from build123d import *

# Parameters (mm, degrees)
F0_W     = 404
F0_H     = 145
F2_DEPTH = 3
F3_D     = 3.3
F3_DEPTH = 8.6
F3_TIP   = 0.9914200214
F1_R     = 1.5
F1_R_2   = 15
F1_R_3   = 1.75
F1_R_4   = 2.5
F1_W     = 55
F1_H     = 15
F4_DEPTH = 25


with BuildPart() as f2:
    # F0 (on Top) → F2 (new body)
    with BuildSketch(Plane.XY):
        with Locations((-14.1859020234, -7.6260944492)):
            Rectangle(F0_W, F0_H)
    extrude(amount=-F2_DEPTH)

    # F3
    with Locations(Plane.XY):
        with Locations((118.573140085, 24.8739055508), (158.573140085, 24.8739055508), (93.573140085, 24.8739055508), (53.573140085, 24.8739055508), (53.573140085, -40.1260944492), (93.573140085, -40.1260944492), (118.573140085, -40.1260944492), (158.573140085, -40.1260944492), (28.573140085, -40.1260944492), (-11.426859915, -40.1260944492), (-11.426859915, 24.8739055508), (28.573140085, 24.8739055508), (-35.926859915, 24.8739055508), (-80.926859915, 24.8739055508), (-80.926859915, -40.1260944492), (-35.926859915, -40.1260944492)):
            Hole(F3_D / 2, depth=F3_DEPTH)
            with Locations((0, 0, -(F3_DEPTH + F3_TIP / 2))):  # 118° drill point
                Cone(0, F3_D / 2, F3_TIP, mode=Mode.SUBTRACT)

    # F1 (on Top) → F4 (cut)
    with BuildSketch(Plane.XY):
        with BuildLine():
            Line((126.323140085, 12.4739055508), (150.823140085, 12.4739055508))
            ThreePointArc((150.823140085, 12.4739055508), (153.6515672098, 13.645478426), (154.823140085, 16.4739055508))
            Line((154.823140085, 16.4739055508), (154.823140085, 33.2739055508))
            ThreePointArc((154.823140085, 33.2739055508), (153.6515672098, 36.1023326755), (150.823140085, 37.2739055508))
            Line((150.823140085, 37.2739055508), (126.323140085, 37.2739055508))
            ThreePointArc((126.323140085, 37.2739055508), (123.4947129603, 36.1023326755), (122.323140085, 33.2739055508))
            Line((122.323140085, 33.2739055508), (122.323140085, 16.4739055508))
            ThreePointArc((122.323140085, 16.4739055508), (123.4947129603, 13.645478426), (126.323140085, 12.4739055508))
        make_face()
        with Locations((158.573140085, 24.8739055508)):
            Circle(F1_R)
        with Locations((118.573140085, 24.8739055508)):
            Circle(F1_R)
        with BuildLine():
            Line((-72.226859915, 10.1239055508), (-44.626859915, 10.1239055508))
            ThreePointArc((-44.626859915, 10.1239055508), (-41.091326009, 11.5883716448), (-39.626859915, 15.1239055508))
            Line((-39.626859915, 15.1239055508), (-39.626859915, 34.6239055508))
            ThreePointArc((-39.626859915, 34.6239055508), (-41.091326009, 38.1594394567), (-44.626859915, 39.6239055508))
            Line((-44.626859915, 39.6239055508), (-72.226859915, 39.6239055508))
            ThreePointArc((-72.226859915, 39.6239055508), (-75.7623938209, 38.1594394567), (-77.226859915, 34.6239055508))
            Line((-77.226859915, 34.6239055508), (-77.226859915, 15.1239055508))
            ThreePointArc((-77.226859915, 15.1239055508), (-75.7623938209, 11.5883716448), (-72.226859915, 10.1239055508))
        make_face()
        with Locations((-35.926859915, 24.8739055508)):
            Circle(F1_R)
        with Locations((-80.926859915, 24.8739055508)):
            Circle(F1_R)
        with BuildLine():
            Line((122.323140085, -31.7260944492), (122.323140085, -48.5260944492))
            ThreePointArc((122.323140085, -48.5260944492), (123.4947129603, -51.354521574), (126.323140085, -52.5260944492))
            Line((126.323140085, -52.5260944492), (150.823140085, -52.5260944492))
            ThreePointArc((150.823140085, -52.5260944492), (153.6515672098, -51.354521574), (154.823140085, -48.5260944492))
            Line((154.823140085, -48.5260944492), (154.823140085, -31.7260944492))
            ThreePointArc((154.823140085, -31.7260944492), (153.6515672098, -28.8976673245), (150.823140085, -27.7260944492))
            Line((150.823140085, -27.7260944492), (126.323140085, -27.7260944492))
            ThreePointArc((126.323140085, -27.7260944492), (123.4947129603, -28.8976673245), (122.323140085, -31.7260944492))
        make_face()
        with Locations((158.573140085, -40.1260944492)):
            Circle(F1_R)
        with Locations((118.573140085, -40.1260944492)):
            Circle(F1_R)
        with BuildLine():
            Line((57.323140085, 33.2739055508), (57.323140085, 16.4739055508))
            ThreePointArc((57.323140085, 16.4739055508), (58.4947129603, 13.645478426), (61.323140085, 12.4739055508))
            Line((61.323140085, 12.4739055508), (85.823140085, 12.4739055508))
            ThreePointArc((85.823140085, 12.4739055508), (88.6515672098, 13.645478426), (89.823140085, 16.4739055508))
            Line((89.823140085, 16.4739055508), (89.823140085, 33.2739055508))
            ThreePointArc((89.823140085, 33.2739055508), (88.6515672098, 36.1023326755), (85.823140085, 37.2739055508))
            Line((85.823140085, 37.2739055508), (61.323140085, 37.2739055508))
            ThreePointArc((61.323140085, 37.2739055508), (58.4947129603, 36.1023326755), (57.323140085, 33.2739055508))
        make_face()
        with Locations((93.573140085, 24.8739055508)):
            Circle(F1_R)
        with Locations((53.573140085, 24.8739055508)):
            Circle(F1_R)
        with BuildLine():
            Line((57.323140085, -31.7260944492), (57.323140085, -48.5260944492))
            ThreePointArc((57.323140085, -48.5260944492), (58.4947129603, -51.354521574), (61.323140085, -52.5260944492))
            Line((61.323140085, -52.5260944492), (85.823140085, -52.5260944492))
            ThreePointArc((85.823140085, -52.5260944492), (88.6515672098, -51.354521574), (89.823140085, -48.5260944492))
            Line((89.823140085, -48.5260944492), (89.823140085, -31.7260944492))
            ThreePointArc((89.823140085, -31.7260944492), (88.6515672098, -28.8976673245), (85.823140085, -27.7260944492))
            Line((85.823140085, -27.7260944492), (61.323140085, -27.7260944492))
            ThreePointArc((61.323140085, -27.7260944492), (58.4947129603, -28.8976673245), (57.323140085, -31.7260944492))
        make_face()
        with Locations((93.573140085, -40.1260944492)):
            Circle(F1_R)
        with Locations((53.573140085, -40.1260944492)):
            Circle(F1_R)
        with BuildLine():
            Line((-7.676859915, 33.2739055508), (-7.676859915, 16.4739055508))
            ThreePointArc((-7.676859915, 16.4739055508), (-6.5052870397, 13.645478426), (-3.676859915, 12.4739055508))
            Line((-3.676859915, 12.4739055508), (20.823140085, 12.4739055508))
            ThreePointArc((20.823140085, 12.4739055508), (23.6515672098, 13.645478426), (24.823140085, 16.4739055508))
            Line((24.823140085, 16.4739055508), (24.823140085, 33.2739055508))
            ThreePointArc((24.823140085, 33.2739055508), (23.6515672098, 36.1023326755), (20.823140085, 37.2739055508))
            Line((20.823140085, 37.2739055508), (-3.676859915, 37.2739055508))
            ThreePointArc((-3.676859915, 37.2739055508), (-6.5052870397, 36.1023326755), (-7.676859915, 33.2739055508))
        make_face()
        with Locations((28.573140085, 24.8739055508)):
            Circle(F1_R)
        with Locations((-11.426859915, 24.8739055508)):
            Circle(F1_R)
        with BuildLine():
            Line((-7.676859915, -31.7260944492), (-7.676859915, -48.5260944492))
            ThreePointArc((-7.676859915, -48.5260944492), (-6.5052870397, -51.354521574), (-3.676859915, -52.5260944492))
            Line((-3.676859915, -52.5260944492), (20.823140085, -52.5260944492))
            ThreePointArc((20.823140085, -52.5260944492), (23.6515672098, -51.354521574), (24.823140085, -48.5260944492))
            Line((24.823140085, -48.5260944492), (24.823140085, -31.7260944492))
            ThreePointArc((24.823140085, -31.7260944492), (23.6515672098, -28.8976673245), (20.823140085, -27.7260944492))
            Line((20.823140085, -27.7260944492), (-3.676859915, -27.7260944492))
            ThreePointArc((-3.676859915, -27.7260944492), (-6.5052870397, -28.8976673245), (-7.676859915, -31.7260944492))
        make_face()
        with Locations((28.573140085, -40.1260944492)):
            Circle(F1_R)
        with Locations((-11.426859915, -40.1260944492)):
            Circle(F1_R)
        with BuildLine():
            Line((-77.226859915, -30.3760944492), (-77.226859915, -49.8760944492))
            ThreePointArc((-77.226859915, -49.8760944492), (-75.7623938209, -53.4116283552), (-72.226859915, -54.8760944492))
            Line((-72.226859915, -54.8760944492), (-44.626859915, -54.8760944492))
            ThreePointArc((-44.626859915, -54.8760944492), (-41.091326009, -53.4116283552), (-39.626859915, -49.8760944492))
            Line((-39.626859915, -49.8760944492), (-39.626859915, -30.3760944492))
            ThreePointArc((-39.626859915, -30.3760944492), (-41.091326009, -26.8405605433), (-44.626859915, -25.3760944492))
            Line((-44.626859915, -25.3760944492), (-72.226859915, -25.3760944492))
            ThreePointArc((-72.226859915, -25.3760944492), (-75.7623938209, -26.8405605433), (-77.226859915, -30.3760944492))
        make_face()
        with Locations((-35.926859915, -40.1260944492)):
            Circle(F1_R)
        with Locations((-80.926859915, -40.1260944492)):
            Circle(F1_R)
        with Locations((-169.1859020234, -40.1260944492)):
            Circle(F1_R_2)
        with Locations((-156.6859020234, -55.1260944492)):
            Circle(F1_R_3)
        with Locations((-181.6859020234, -25.1260944492)):
            Circle(F1_R_3)
        with Locations((-188.1859020234, -71.9773098826)):
            Circle(F1_R_4)
        with BuildLine():
            Line((-131.9859020234, -35.8176724643), (-131.9859020234, -44.4345164341))
            ThreePointArc((-131.9859020234, -44.4345164341), (-125.1859020234, -48.1760944492), (-118.3859020234, -44.4345164341))
            Line((-118.3859020234, -44.4345164341), (-118.3859020234, -35.8176724643))
            ThreePointArc((-118.3859020234, -35.8176724643), (-125.1859020234, -32.0760944492), (-131.9859020234, -35.8176724643))
        make_face()
        with Locations((-183.6481976509, 24.6848849975)):
            Rectangle(F1_W, F1_H)
        with Locations((-123.6481976509, 24.6848849975)):
            Rectangle(F1_W, F1_H)
    extrude(amount=-F4_DEPTH, mode=Mode.SUBTRACT)


solid = f2.part
Verification items for the finished model (mm, model axes). Give positions to 0.01 mm unless a question says otherwise; leave off trailing zeros. Loops run counter-clockwise (first coordinate to the right, second up) from the corner with the lowest first, then second, coordinate; pieces in that order, holes last.
1) Draft check along X on faces 1 (the cylindrical face through (-184.17, -39.47, -1.48)), 2 (the flat face through (-17, -7, -3)). Enter one of: pulls with the +X half, pulls with the -X half, needs draft (parallel to the pull), parting line crosses it, or undercut.
2) Thickness scan on line 1 along Y through (x, z) = (-46.5, -1.5); line 2 along Y through (x, z) = (-166.5, -1.7); line 3 along Y through (x, z) = (-133, -2.8). Record the ranges inside material, lowest first.
3) Sectioned sample at A-A, the plane x = -122. Enter the section's corners in (y, z), then the cut area to 3 significant figures.
4) Sectioned sample at B-B, the plane z = -1.7. Count the separate pieces of the cut face and the enclosed holes in it, then the cut area to 3 significant figures.
Answers:
1. face 1: undercut
1. face 2: needs draft
2. line 1: y = -80.13 to -54.88, -25.38 to 10.12, 39.62 to 64.87
2. line 2: y = -80.13 to -54.88, -25.37 to 17.18, 32.18 to 64.87
2. line 3: y = -80.13 to 17.18, 32.18 to 64.87
3. outline: (-80.13, -3) - (-47.52, -3) - (-47.52, 0) - (-80.13, 0) - close; (-32.73, -3) - (17.18, -3) - (17.18, 0) - (-32.73, 0) - close; (32.18, -3) - (64.87, -3) - (64.87, 0) - (32.18, 0) - close
3. area: 346 mm2
4. separate pieces: 1
4. enclosed holes: 31
4. area: 48,900 mm2
